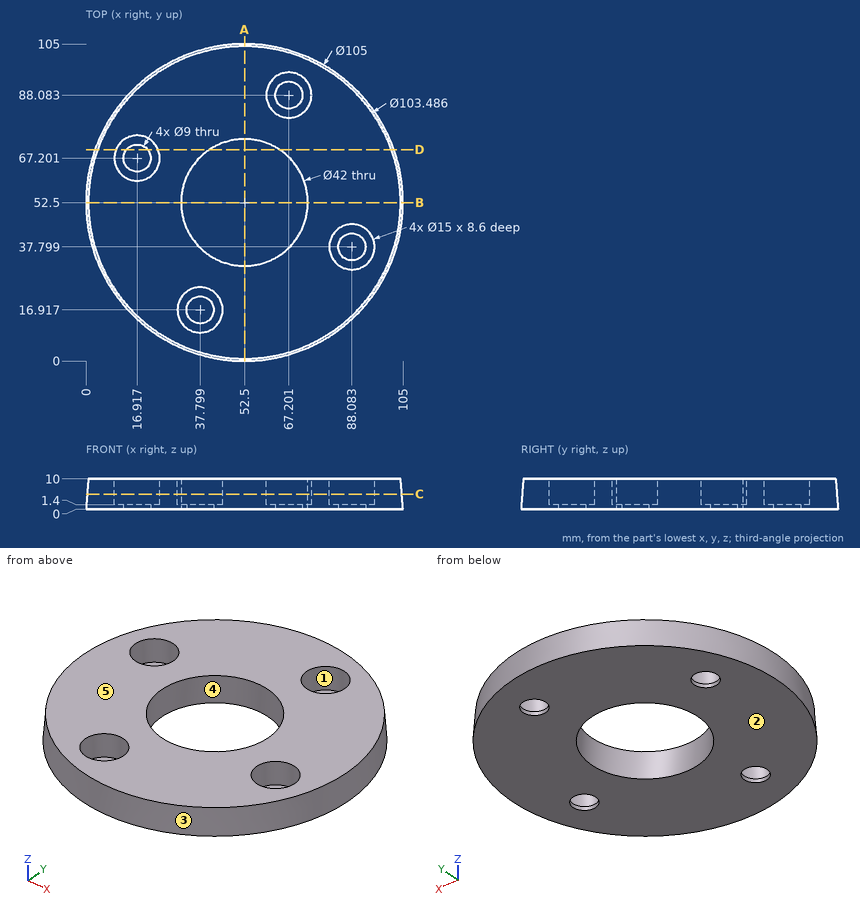
Study the drawing (mm; zero at the part's minimum x, y, z) and answer. A direction names the side the tool comes from. Give positions to 0.01 mm unless a question says otherwise; leave off trailing zeros. Order: outer loops, then holes, each group sorted by start corner. A loop starts at its lowest first (then second) coordinate and runs counter-clockwise, first axis right, second up. Notation, with made-up numbers: (-11, -11.5) - (10, -11.5) arc R21 ccw to (10, 4.5) - close; hole circle Ø1 at (-13, 40.25). An arc over 180 degrees is marked (long way). Answer as CSV lines item,"result". Start each with the question number.
Q1. For the marked faces 1 and 2, determine the directions among +Z, -Z, +X, -X, +Y, -Y from which every point of the face is accessible in a straight line to the end or side of a thin tool.
Q2. The part is cut by section C-C (z = 5). Write down the section's boundary in (x, y).
Q3. Find the intervals of material crossed by L1, parallel to Y at x = 63.5, z = 7.25 (1 decimal); L2, parallel to Z at x = 66.5, y = 83; L3, parallel to Y at x = 21, z = 3 (1 decimal), in increasing order. Write a range as [from, to].
Q4. The mould has two halves that part along Y. Classify the marked faces 3, 4 and 5: +Y half, -Y half, draft (parallel to the pull), parting line (faces both ways), or undercut.
Q5. Given pin 1 Ø7 at (x, y) = (37.8, 16.92) entering from -Z; pin 2 Ø6 at (x, z) = (21.5, 5) entering from +Y; pin 3 Ø7.5 at (x, y) = (19, 70) entering from +Z; pin 4 Ø6 at (x, z) = (36.5, 6) entering from -Y, each flat-ended and moving along its own axis, determine where each tip first touches the part or whether it passes through.
Q6. The part is cut by section D-D (y = 70). Give the number of separate pieces and of enclosed holes in the cut face, then the cut area to 3 significant figures.
Q7. The part is cut by section A-A (x = 52.5). Write down the section's boundary in (y, z).
Check result:
1,face 1,"+Z"
1,face 2,"-Z, +X, -X, +Y, -Y"
2,outline,"circle Ø104.24 at (52.5, 52.5); hole circle Ø15 at (16.92, 67.2); hole circle Ø15 at (37.8, 16.92); hole circle Ø42 at (52.5, 52.5); hole circle Ø15 at (67.2, 88.08); hole circle Ø15 at (88.08, 37.8)"
3,L1,"y = [1.7, 34.6], [70.4, 81.6], [94.6, 103.3]"
3,L2,"z = [0, 1.4]"
3,L3,"y = [10.8, 60.9], [73.5, 94.2]"
4,face 3,"parting line"
4,face 4,"undercut"
4,face 5,"draft"
5,pin 1,"passes through"
5,pin 2,"stops at y = 96.48"
5,pin 3,"stops at z = 1.4"
5,pin 4,"stops at y = 2.07"
6,separate pieces,"3"
6,enclosed holes,"0"
6,area,"620 mm²"
7,outline,"(0, 0) - (31.5, 0) - (31.5, 10) - (0.76, 10) - close; (73.5, 0) - (105, 0) - (104.24, 10) - (73.5, 10) - close"
